The model under review builds one solid part; all positions refer to its coordinate system, in mm. A direction names the side the tool comes from. Round coordinates to 2 decimals unless told otherwise and drop trailing zeros. Order: outer loops, then holes, each group sorted by start corner. A loop starts at its lowest first (then second) coordinate and runs counter-clockwise, first axis right, second up. Notation, with made-up numbers: (8, 89.5) - (20, 89.5) arc R21 ccw to (20, 103.5) - close; hole circle Ø7 at (61.25, 56.25). An arc over 180 degrees is marked (long way). One line per question, with ' | ' between items. Start each with the question number.
Item 1: Draft analysis for pull direction X (two halves, no side actions). For faces 3 (the face through (0, 795, 0)), 4 (the face through (-25, 795, 63)), 5 (the face through (0, 795, 3)), state which applies: +X half, -X half, draft (parallel to the pull), parting line (faces both ways), or undercut.
Item 2: Insertion check: pin 1 Ø10 at (x, y) = (14.5, 768) entering from +Z; pin 2 Ø0.9 at (y, z) = (1431.5, 1.5) entering from -X; pin 3 Ø8 at (y, z) = (542, 15.5) entering from -X; pin 4 Ø5.5 at (x, y) = (0, 25) entering from +Z. Each pin has a flat end and moves straight along its axis. Give the tip position at first contact, or say it passes through.
Item 3: Add section A-A on y = 1195. State the section outline as (x, z) points, and give its area (3 significant figures).
Item 4: For L1, parallel to Y at x = 23.45, z = 15.5; L2, parallel to X at y = 749, z = 8.5; L3, parallel to Z at x = 3.5, y = 1040, list the stretches that pass through material, from the lowest coordinate up. Write a range as [from, to].
Item 5: Tool access review of faces 1 (the face through (-22, 795, 61)), 2 (the face through (-24, 1613, 37)): name each direction out of +Z, -Z, +X, -X, +Y, -Y from which nothing blocks a thin tool from reaching the whole face with its end or side.
from build123d import *

# Parameters (mm, degrees)
BASE_FLANGE1_DEPTH = 1613
CUT_EXTRUDE1_REACH = 1620.23
FILLET1_R          = 3
CUT_EXTRUDE2_REACH = 1620.23
SKETCH7_R          = 4.5
LPATTERN1_COUNT    = 4
LPATTERN1_PITCH    = 529
CUT_EXTRUDE3_REACH = 1620.23
SKETCH8_R          = 3.25
CUT_EXTRUDE4_REACH = 1619.431
CUT_EXTRUDE5_REACH = 1619.431
SKETCH10_R         = 4.5
LPATTERN2_COUNT    = 3
LPATTERN2_PITCH    = 529
CUT_EXTRUDE6_REACH = 1619.431
SKETCH11_R         = 4.5


# Sheet-metal steps are written as plain solids
with BuildPart() as part:
    # Sketch1 → Base-Flange1 (new body)
    with BuildSketch(Plane(origin=(0, 0, 0), x_dir=(1, 0, 0), z_dir=(0, 1, 0))):
        with BuildLine():
            Line((-25, -120), (-25, -4.5))
            ThreePointArc((-25, -4.5), (-23.681980515, -1.318019485), (-20.5, 0))
            Line((-20.5, 0), (20.5, 0))
            ThreePointArc((20.5, 0), (23.681980515, -1.318019485), (25, -4.5))
            Line((25, -4.5), (25, -25))
            Line((25, -25), (22, -25))
            Line((22, -25), (22, -4.5))
            ThreePointArc((22, -4.5), (21.560660172, -3.439339828), (20.5, -3))
            Line((20.5, -3), (-20.5, -3))
            ThreePointArc((-20.5, -3), (-21.560660172, -3.439339828), (-22, -4.5))
            Line((-22, -4.5), (-22, -120))
            Line((-22, -120), (-25, -120))
        make_face()
    extrude(amount=BASE_FLANGE1_DEPTH)

    # Sketch6 → Cut-Extrude1 (cut, up to next)
    with BuildSketch(Plane.ZY.offset(25), mode=Mode.PRIVATE) as cut_extrude1_sk1:
        with BuildLine():
            Line((14.5, 16.25), (22.5, 16.25))
            ThreePointArc((22.5, 16.25), (25.75, 13), (22.5, 9.75))
            Line((22.5, 9.75), (14.5, 9.75))
            ThreePointArc((14.5, 9.75), (11.25, 13), (14.5, 16.25))
        make_face()
    cut_extrude1_tool1 = extrude(cut_extrude1_sk1.sketch, amount=-CUT_EXTRUDE1_REACH, mode=Mode.PRIVATE) & part.part
    cut_extrude1 = cut_extrude1_tool1.solids().sort_by_distance((-25, 13, 18.5))[0]
    add(cut_extrude1, mode=Mode.SUBTRACT)

    # Fillet1
    fillet1_edges = [part.edges().sort_by_distance(p)[0] for p in [
        (23.5, 0, 25),
        (-23.5, 0, 120),
        (23.5, 1613, 25),
        (-23.5, 1613, 120),
    ]]
    fillet(fillet1_edges, radius=FILLET1_R)

    # Sketch7 → Cut-Extrude2 (cut, up to next)
    with BuildSketch(Plane(origin=(25, 0, 0), x_dir=(0, 0, -1), z_dir=(1, 0, 0)), mode=Mode.PRIVATE) as cut_extrude2_sk1:
        with Locations((-15.5, 13)):
            Circle(SKETCH7_R)
    cut_extrude2_tool1 = extrude(cut_extrude2_sk1.sketch, amount=-CUT_EXTRUDE2_REACH, mode=Mode.PRIVATE) & part.part
    cut_extrude2 = cut_extrude2_tool1.solids().sort_by_distance((25, 13, 15.5))[0]
    add(cut_extrude2, mode=Mode.SUBTRACT)

    # LPattern1: Cut-Extrude1, Cut-Extrude2 ×4
    with Locations(*[(0, i * LPATTERN1_PITCH, 0) for i in range(1, LPATTERN1_COUNT)]):
        add(cut_extrude1, mode=Mode.SUBTRACT)
        add(cut_extrude2, mode=Mode.SUBTRACT)

    # Sketch8 → Cut-Extrude3 (cut, up to next)
    with BuildSketch(Plane.ZY.offset(25), mode=Mode.PRIVATE) as cut_extrude3_sk1:
        with Locations((50.716371709, 1515.981333294)):
            Circle(SKETCH8_R)
    cut_extrude3_tool1 = extrude(cut_extrude3_sk1.sketch, amount=-CUT_EXTRUDE3_REACH, mode=Mode.PRIVATE) & part.part
    # Sketch8 → Cut-Extrude3 (cut, up to next)
    with BuildSketch(Plane.ZY.offset(25), mode=Mode.PRIVATE) as cut_extrude3_sk2:
        with Locations((89.283628291, 1470.018666706)):
            Circle(SKETCH8_R)
    cut_extrude3_tool2 = extrude(cut_extrude3_sk2.sketch, amount=-CUT_EXTRUDE3_REACH, mode=Mode.PRIVATE) & part.part
    add(cut_extrude3_tool1.solids().sort_by_distance((-25, 1515.981333, 50.716372))[0], mode=Mode.SUBTRACT)
    add(cut_extrude3_tool2.solids().sort_by_distance((-25, 1470.018667, 89.283628))[0], mode=Mode.SUBTRACT)

    # Sketch9 → Cut-Extrude4 (cut, up to next)
    with BuildSketch(Plane.XY.offset(3), mode=Mode.PRIVATE) as cut_extrude4_sk1:
        with BuildLine():
            Line((-16.5, 1417), (-16.5, 1447))
            ThreePointArc((-16.5, 1447), (-1.5, 1462), (13.5, 1447))
            Line((13.5, 1447), (13.5, 1417))
            ThreePointArc((13.5, 1417), (-1.5, 1402), (-16.5, 1417))
        make_face()
    cut_extrude4_tool1 = extrude(cut_extrude4_sk1.sketch, amount=-CUT_EXTRUDE4_REACH, mode=Mode.PRIVATE) & part.part
    add(cut_extrude4_tool1.solids().sort_by_distance((-1.5, 1432, 3))[0], mode=Mode.SUBTRACT)

    # Sketch10 → Cut-Extrude5 (cut, up to next)
    with BuildSketch(Plane.XY.offset(3), mode=Mode.PRIVATE) as cut_extrude5_sk1:
        with Locations((0, 25)):
            Circle(SKETCH10_R)
    cut_extrude5_tool1 = extrude(cut_extrude5_sk1.sketch, amount=-CUT_EXTRUDE5_REACH, mode=Mode.PRIVATE) & part.part
    cut_extrude5 = cut_extrude5_tool1.solids().sort_by_distance((0, 25, 3))[0]
    add(cut_extrude5, mode=Mode.SUBTRACT)

    # LPattern2: Cut-Extrude5 ×3
    with Locations(*[(0, i * LPATTERN2_PITCH, 0) for i in range(1, LPATTERN2_COUNT)]):
        add(cut_extrude5, mode=Mode.SUBTRACT)

    # Sketch11 → Cut-Extrude6 (cut, up to next)
    with BuildSketch(Plane.XY.offset(3), mode=Mode.PRIVATE) as cut_extrude6_sk1:
        with Locations((0, 1588)):
            Circle(SKETCH11_R)
    cut_extrude6_tool1 = extrude(cut_extrude6_sk1.sketch, amount=-CUT_EXTRUDE6_REACH, mode=Mode.PRIVATE) & part.part
    add(cut_extrude6_tool1.solids().sort_by_distance((0, 1588, 3))[0], mode=Mode.SUBTRACT)


solid = part.part
Determined:
1) face 3: draft | face 4: -X half | face 5: undercut
2) pin 1: z = 3 | pin 2: x = -24.21 | pin 3: x = -25 | pin 4: through
3) outline: (-25, 4.5) arc R4.5 ccw to (-20.5, 0) - (20.5, 0) arc R4.5 ccw to (25, 4.5) - (25, 25) - (22, 25) - (22, 4.5) arc R1.5 cw to (20.5, 3) - (-20.5, 3) arc R1.5 cw to (-22, 4.5) - (-22, 120) - (-25, 120) - close | area: 559 mm2
4) L1: [0, 8.5], [17.5, 537.5], [546.5, 1066.5], [1075.5, 1595.5], [1604.5, 1613] | L2: [-25, -22], [22, 25] | L3: [0, 3]
5) face 1: +Z, +Y, -Y | face 2: +Z, -Z, +X, -X, +Y
